```python
from build123d import *

# Parameters (mm, degrees)
SKETCH_1_W          = 23
SKETCH_1_H          = 23
SKETCH_1_W_2        = 13
SKETCH_1_H_2        = 13
EXTRUDE_1_DEPTH     = 35
SKETCH_2_R          = 1.65
CUT_EXTRUDE_1_DEPTH = 34
SKETCH_4_W          = 23
SKETCH_4_H          = 23
SKETCH_4_R          = 3
EXTRUDE_2_DEPTH     = 3.5
SKETCH_5_W          = 23
SKETCH_5_H          = 23
SKETCH_5_W_2        = 13
SKETCH_5_H_2        = 13
EXTRUDE_1_2_DEPTH   = 54
SKETCH_6_R          = 1.65
CUT_EXTRUDE_2_DEPTH = 39
SKETCH_7_W          = 13
SKETCH_7_H          = 13
CUT_EXTRUDE_3_DEPTH = 13
CHAMFER_1_SIZE      = 3
SKETCH_8_W          = 80.5
SKETCH_8_H          = 35
CUT_EXTRUDE_4_DEPTH = 11.5
EXTRUDE_3_DEPTH     = 6.5
FILLET_1_R          = 10
FILLET_2_R          = 10
SKETCH_10_R         = 1.65
CUT_EXTRUDE_5_DEPTH = 28.5
CHAMFER_4_SIZE      = 3
CHAMFER_START       = 6.5
CHAMFER_5_DEPTH     = 11.5
SKETCH_11_W         = 10
SKETCH_11_H         = 13
EXTRUDE_4_DEPTH     = 10
CHAMFER_9_SIZE      = 5
CHAMFER_10_SIZE     = 5
CHAMFER_11_SIZE     = 10
CHAMFER_12_SIZE     = 10
CHAMFER_13_SIZE     = 1.5
CHAMFER_14_SIZE     = 1.5
SKETCH_12_W         = 99.580162389
SKETCH_12_H         = 41.70081518
CUT_EXTRUDE_6_DEPTH = 35


with BuildPart() as part:
    # 草图1 → Extrude 1 (new body)
    with BuildSketch(Plane.XY):
        with Locations((6.5, 6.5)):
            Rectangle(SKETCH_1_W, SKETCH_1_H)
        with Locations((6.5, 6.5)):
            Rectangle(SKETCH_1_W_2, SKETCH_1_H_2, mode=Mode.SUBTRACT)
    extrude(amount=EXTRUDE_1_DEPTH)

    # 草图2 → 切除-拉伸1 (cut)
    with BuildSketch(Plane.XZ.offset(5)):
        with Locations(Location((6.5, 25, 0), (0, 0, 270))):
            Circle(SKETCH_2_R)
    extrude(amount=-CUT_EXTRUDE_1_DEPTH, mode=Mode.SUBTRACT)

    # 草图4 → 凸台-拉伸2 (add)
    with BuildSketch(Plane(origin=(18, 0, 0), x_dir=(0, 0, -1), z_dir=(1, 0, 0))):
        with Locations((-11.5, 6.5)):
            Rectangle(SKETCH_4_W, SKETCH_4_H)
        with Locations(Location((-11.5, 6.5, 0), (0, 0, 90))):
            Circle(SKETCH_4_R, mode=Mode.SUBTRACT)
    extrude(amount=EXTRUDE_2_DEPTH)

    # 草图5 → Extrude 1 2 (add)
    with BuildSketch(Plane(origin=(21.5, 0, 0), x_dir=(0, 0, -1), z_dir=(1, 0, 0))):
        with Locations((-11.5, 6.5)):
            Rectangle(SKETCH_5_W, SKETCH_5_H)
        with Locations((-11.5, 6.5)):
            Rectangle(SKETCH_5_W_2, SKETCH_5_H_2, mode=Mode.SUBTRACT)
    extrude(amount=EXTRUDE_1_2_DEPTH)

    # 草图6 → 切除-拉伸2 (cut)
    with BuildSketch(Plane(origin=(0, 18, 0), x_dir=(1, 0, 0), z_dir=(0, 1, 0))):
        with Locations(Location((65.5, -11.5, 0), (0, 0, 270))):
            Circle(SKETCH_6_R)
    extrude(amount=-CUT_EXTRUDE_2_DEPTH, mode=Mode.SUBTRACT)

    # 草图7 → 切除-拉伸3 (cut)
    with BuildSketch(Plane(origin=(21.5, 0, 0), x_dir=(0, 0, -1), z_dir=(1, 0, 0))):
        with Locations((-11.5, 6.5)):
            Rectangle(SKETCH_7_W, SKETCH_7_H)
    extrude(amount=-CUT_EXTRUDE_3_DEPTH, mode=Mode.SUBTRACT)

    # 倒角1
    chamfer_1_edges = [part.edges().sort_by_distance(p)[0] for p in [
        (13, 6.5, 18),
    ]]
    chamfer(chamfer_1_edges, length=CHAMFER_1_SIZE)

    # 草图8 → 切除-拉伸4 (cut)
    with BuildSketch(Plane.XZ.offset(5)):
        with Locations((35.25, 17.5)):
            Rectangle(SKETCH_8_W, SKETCH_8_H)
    extrude(amount=-CUT_EXTRUDE_4_DEPTH, mode=Mode.SUBTRACT)

    # 草图9 → 凸台-拉伸3 (add)
    with BuildSketch(Plane.XZ.offset(-13)):
        Polygon((13, 5), (0, 16), (0, 0), (13, 0), align=None)
    extrude(amount=EXTRUDE_3_DEPTH)

    # 圆角1
    fillet_1_edges = [part.edges().sort_by_distance(p)[0] for p in [
        (-5, 12.25, 0),
    ]]
    fillet(fillet_1_edges, radius=FILLET_1_R)

    # 圆角2
    fillet_2_edges = [part.edges().sort_by_distance(p)[0] for p in [
        (18, 12.25, 23),
    ]]
    fillet(fillet_2_edges, radius=FILLET_2_R)

    # 草图10 → 切除-拉伸5 (cut)
    with BuildSketch(Plane.XZ.offset(-6.5)):
        with Locations(Location((2, 7, 0), (0, 0, 270))):
            Circle(SKETCH_10_R)
        with Locations(Location((18, 23, 0), (0, 0, 270))):
            Circle(SKETCH_10_R)
    extrude(amount=-CUT_EXTRUDE_5_DEPTH, mode=Mode.SUBTRACT)

    # 倒角4
    chamfer_4_edges = [part.edges().sort_by_distance(p)[0] for p in [
        (75.5, 18, 11.5),
        (6.5, 18, 35),
    ]]
    chamfer(chamfer_4_edges, length=CHAMFER_4_SIZE)

    # 倒角5: read off the stored shape, not the designer's step
    # 倒角5 outline → 倒角5 (cut)
    with BuildSketch(Plane(origin=(0, 0, 0), x_dir=(1, 0, 0), z_dir=(0, 1, 0)).offset(CHAMFER_START)):
        Polygon((72.5, 0), (75.5, -3), (75.5, 0), align=None)
        Polygon((-5, -35), (-2, -35), (-5, -32), align=None)
        with BuildLine():
            ThreePointArc((18, -33), (18.007410169, -32.615099398), (18.029629695, -32.230769231))
            Line((18.029629695, -32.230769231), (15.038518603, -35))
            Line((15.038518603, -35), (18, -35))
            Line((18, -35), (18, -33))
        make_face()
        Polygon((75.5, -20), (72.5, -23), (75.5, -23), align=None)
    extrude(amount=CHAMFER_5_DEPTH, mode=Mode.SUBTRACT)


with BuildPart() as body_2:
    # Split Bodies 1: the piece on the far side of the plane
    add(part.part)
    split(bisect_by=Plane.YZ.offset(50.5), keep=Keep.BOTTOM)


with BuildPart() as part_1:
    add(part.part)

    # Split Bodies 1
    split(bisect_by=Plane.YZ.offset(50.5), keep=Keep.TOP)


with BuildPart() as part_2:
    # Move Body 1: read off the stored shape, not the designer's step
    # Move Body 1: moved
    add(part_1.part.moved(Location((0, -10, 0))))

    # Combine 1: union body 2
    add(body_2.part)

    # 草图11 → 凸台-拉伸4 (add)
    with BuildSketch(Plane.XZ.offset(-13)):
        with Locations((45.5, 11.5)):
            Rectangle(SKETCH_11_W, SKETCH_11_H)
    extrude(amount=EXTRUDE_4_DEPTH)

    # 倒角9
    chamfer_9_edges = [part_2.edges().sort_by_distance(p)[0] for p in [
        (50.5, 18, 11.5),
    ]]
    chamfer(chamfer_9_edges, length=CHAMFER_9_SIZE)

    # 倒角10
    chamfer_10_edges = [part_2.edges().sort_by_distance(p)[0] for p in [
        (50.5, 8, 11.5),
    ]]
    chamfer(chamfer_10_edges, length=CHAMFER_10_SIZE - 0.0001)  # a hair under: the kernel refuses the full size

    # 倒角11
    # the kernel refuses this chamfer: 10 mm, written as the material it adds along each edge
    with BuildSketch(Plane(origin=(50.5, 6.5, 30.71682988), x_dir=(-1, 0, 0), z_dir=(0, 0, -1))) as chamfer_11_piece_1_section:
        Polygon((CHAMFER_11_SIZE, 0), (0, -CHAMFER_11_SIZE), (0, 0), align=None)
    chamfer_11_piece_1 = extrude(amount=30.71682988, mode=Mode.PRIVATE)
    chamfer_11_piece_1 = split(chamfer_11_piece_1, bisect_by=Plane(origin=(50.5, -3.5, 30.71682988), z_dir=(0, 1, 0)), keep=Keep.TOP, mode=Mode.PRIVATE)
    chamfer_11_piece_1 = split(chamfer_11_piece_1, bisect_by=Plane(origin=(50.5, 6.5, 23), z_dir=(0, 0, -1)), keep=Keep.TOP, mode=Mode.PRIVATE)
    chamfer_11_piece_1 = split(chamfer_11_piece_1, bisect_by=Plane(origin=(50.5, 6.5, 18), z_dir=(0, 0, 1)), keep=Keep.TOP, mode=Mode.PRIVATE)
    add(chamfer_11_piece_1)
    with BuildSketch(Plane(origin=(50.5, 6.5, 5), x_dir=(-1, 0, 0), z_dir=(0, 0, -1))) as chamfer_11_piece_2_section:
        Polygon((CHAMFER_11_SIZE, 0), (0, -CHAMFER_11_SIZE), (0, 0), align=None)
    chamfer_11_piece_2 = extrude(amount=5, mode=Mode.PRIVATE)
    chamfer_11_piece_2 = split(chamfer_11_piece_2, bisect_by=Plane(origin=(50.5, -3.5, 5), z_dir=(0, 1, 0)), keep=Keep.TOP, mode=Mode.PRIVATE)
    add(chamfer_11_piece_2)
    with BuildSketch(Plane(origin=(50.5, 6.5, 23), x_dir=(-1, 0, 0), z_dir=(0, 0, -1))) as chamfer_11_piece_3_section:
        Polygon((CHAMFER_11_SIZE, 0), (0, -CHAMFER_11_SIZE), (0, 0), align=None)
    chamfer_11_piece_3 = extrude(amount=5, mode=Mode.PRIVATE)
    chamfer_11_piece_3 = split(chamfer_11_piece_3, bisect_by=Plane(origin=(50.5, -3.5, 23), z_dir=(0, 1, 0)), keep=Keep.TOP, mode=Mode.PRIVATE)
    add(chamfer_11_piece_3)
    with BuildSketch(Plane(origin=(50.5, 6.5, 23), x_dir=(-1, 0, 0), z_dir=(0, 0, -1))) as chamfer_11_piece_4_section:
        Polygon((CHAMFER_11_SIZE, 0), (0, -CHAMFER_11_SIZE), (0, 0), align=None)
    chamfer_11_piece_4 = extrude(amount=30.71682988, mode=Mode.PRIVATE)
    chamfer_11_piece_4 = split(chamfer_11_piece_4, bisect_by=Plane(origin=(50.5, 6.5, 0), z_dir=(0, 0, 1)), keep=Keep.TOP, mode=Mode.PRIVATE)
    chamfer_11_piece_4 = split(chamfer_11_piece_4, bisect_by=Plane(origin=(50.5, -3.5, 23), z_dir=(0, 1, 0)), keep=Keep.TOP, mode=Mode.PRIVATE)
    chamfer_11_piece_4 = split(chamfer_11_piece_4, bisect_by=Plane(origin=(50.5, 6.5, 5), z_dir=(0, 0, -1)), keep=Keep.TOP, mode=Mode.PRIVATE)
    add(chamfer_11_piece_4)

    # 倒角12
    # the kernel refuses this chamfer: 10 mm, written as the material it takes off along each edge
    with BuildSketch(Plane(origin=(40.5, 3, 5), x_dir=(1, 0, 0), z_dir=(0, 0, 1))) as chamfer_12_piece_1:
        Polygon((CHAMFER_12_SIZE, 0), (0, CHAMFER_12_SIZE), (0, 0), align=None)
    extrude(amount=13, mode=Mode.SUBTRACT)

    # 倒角13
    chamfer_13_edges = [part_2.edges().sort_by_distance(p)[0] for p in [
        (-5, 18, 21),
        (-2.071067812, 18, 2.928932188),
        (25.25, 18, 0),
        (21.291796068, 18, 25.583801513),
        (36.75, 18, 23),
    ]]
    chamfer(chamfer_13_edges, length=CHAMFER_13_SIZE)

    # 倒角14
    chamfer_14_edges = [part_2.edges().sort_by_distance(p)[0] for p in [
        (48.75, 14.75, 0),
        (50.5, 12.99995, 0),
        (52.99995, 10.49995, 0),
        (63.99995, 8, 0),
        (48.75, 14.75, 23),
        (50.5, 12.99995, 23),
        (52.99995, 10.49995, 23),
        (63.99995, 8, 23),
    ]]
    chamfer(chamfer_14_edges, length=CHAMFER_14_SIZE)

    # 镜向1: part across face


with BuildPart() as part_3:
    add(part_2.part)
    add(part_2.part.mirror(Plane(origin=(39.29455316, 7.74366918, 0), x_dir=(1, 0, 0), z_dir=(0, 0, -1))))

    # 草图12 → 切除-拉伸6 (cut)
    with BuildSketch(Plane.XY.offset(35)):
        with Locations((40.094907988, 6.821209465)):
            Rectangle(SKETCH_12_W, SKETCH_12_H)
    extrude(amount=-CUT_EXTRUDE_6_DEPTH, mode=Mode.SUBTRACT)


solid = part_3.part
```
Geometry: final body of the model. Coordinates: model frame, mm. A direction names the side the tool comes from. Round coordinates to 2 decimals unless told otherwise and drop trailing zeros. Order: outer loops, then holes, each group sorted by start corner. A loop starts at its lowest first (then second) coordinate and runs counter-clockwise, first axis right, second up. Notation, with made-up numbers: M 46.25,60 L 56.25,60 A16 cw 56.25,85 Z; hole C 73,27 d6. An arc over 180 degrees is marked long. Use one line per item in the form item = value. Start each with the question number.
Q1. Access query for faces 1 (the face through (62, 8, -12)), 2 (the face through (6.591, 9.796, -10.423)), 3 (the face through (36.6, 17.2, -22.3)), 4 (the face through (14, 10, -20)). Directions: +Z, -Z, +X, -X, +Y, -Y. A direction counts if a zero-diameter tool reaches every point of the face in a straight line with its end or side. Return the directions, or none.
Q2. Cut plane A-A (y = 1.75). Return loops of the section in (x, z).
Q3. Material intervals for line 1 (Z direction, x = 57.5, y = 0.5); line 2 (Y direction, x = 1, z = -8.5); line 3 (X direction, y = 15.3, z = -25), sorted ascending. Write a range as [from, to].
Q4. Cut plane B-B (x = 65.5). Return loops of the section in (y, z).
Q5. Mould query, pull axis Z, two halves, no side actions, for faces 5 (the face through (24, 6.5, -23)), 6 (the face through (47.497, 14.927, -22.26)), 7 (the face through (18.07, 12.17, -24.65)). Classes: +Z half, -Z half, draft (parallel to the pull), parting line (faces both ways), or undercut.
Q6. Pin query (flat end, axial travel): pin 1 Ø10.5 at (x, z) = (28, -15) entering from -Y; pin 2 Ø2.5 at (x, z) = (18, -23) entering from +Y; pin 3 Ø8 at (x, y) = (39.5, 4) entering from -Z; pin 4 Ø8.5 at (x, z) = (65, -11.5) entering from +Y. Return the tip coordinate at first contact, or that it passes through.
Geometry results:
q1.face_1 = +Z, -Z, +X, +Y
q1.face_2 = -Z, -Y
q1.face_3 = -Z, +X, +Y
q1.face_4 = -Y
q2.outline = M 45.25,-23 L 72.5,-23 L 75.5,-20 L 75.5,-18 L 45.25,-18 Z; M 45.25,-5 L 75.5,-5 L 75.5,-3 L 72.5,0 L 45.25,0 Z
q3.line_1 = [-23, -18], [-5, 0]
q3.line_2 = [6.5, 18]
q3.line_3 = [-5, 4.85], [8.15, 22]
q4.outline = M -3.5,-23 L 6.5,-23 L 8,-21.5 L 8,-13.15 L 3,-13.15 L 3,-18 L -3.5,-18 Z; M -3.5,-5 L 3,-5 L 3,-9.85 L 8,-9.85 L 8,-1.5 L 6.5,0 L -3.5,0 Z
q5.face_5 = draft
q5.face_6 = -Z half
q5.face_7 = undercut
q6.pin_1 = 6.5
q6.pin_2 = through
q6.pin_3 = -23
q6.pin_4 = 8
